from build123d import *

# Parameters (mm, degrees)
BOSS_EXTRU_1_DEPTH             = 4
BOSS_EXTRU_1_DEPTH_BACK        = 4
ESQUISSE3_R                    = 2
ENL_V_MAT_EXTRU_1_DEPTH        = 5
ENL_V_MAT_EXTRU_1_DEPTH_BACK   = 5
BOSS_EXTRU_2_REACH             = 6
BOSS_EXTRU_2_DIRECTION_2_REACH = 6
ENL_V_START                    = -4
ESQUISSE4_W                    = 60
ESQUISSE4_H                    = 3.5
ENL_V_MAT_EXTRU_2_DEPTH        = 5
ENL_V_START_2                  = 9.713229
ESQUISSE7_R                    = 1.5
ENL_V_MAT_EXTRU_4_DEPTH        = 6.063229
CONG_1_R                       = 10
CONG_2_R                       = 2


with BuildPart() as part:
    # Esquisse1 → Boss.-Extru.1 (new body, two sides)
    with BuildSketch(Plane.XY) as boss_extru_1_sk:
        Polygon((-18.056919343, 0.131274222), (-15.479170984, -5.286770941), (18.771312817, -5.286770941), (21.159805355, 1.060426821), (3, 16.8), (-3, 16.8), align=None)
    extrude(amount=BOSS_EXTRU_1_DEPTH)
    extrude(boss_extru_1_sk.sketch, amount=-BOSS_EXTRU_1_DEPTH_BACK)

    # Esquisse3 → Enlèv. mat.-Extru.1 (cut, two sides)
    with BuildSketch(Plane.XY) as enl_v_mat_extru_1_sk:
        with Locations((0, 10.8)):
            Circle(ESQUISSE3_R)
        with Locations((-11.35, 0)):
            Circle(ESQUISSE3_R)
        with Locations((14.35, 0)):
            Circle(ESQUISSE3_R)
    extrude(amount=ENL_V_MAT_EXTRU_1_DEPTH, mode=Mode.SUBTRACT)
    extrude(enl_v_mat_extru_1_sk.sketch, amount=-ENL_V_MAT_EXTRU_1_DEPTH_BACK, mode=Mode.SUBTRACT)

    # Boss.-Extru.2: up to this face of the body (flat: up to its plane)
    boss_extru_2_end = Plane(part.part.faces().sort_by_distance((1.373128785, 3.366991502, 4))[0])
    # Esquisse6 → Boss.-Extru.2 (add, up to the picked face)
    with BuildSketch(Plane.XY, mode=Mode.PRIVATE) as boss_extru_2_sk1:
        Polygon((-9.401505424, 9.713229059), (-30, 9.713229059), (-30, -5.286770941), (-15.479170984, -5.286770941), (-18.056919343, 0.131274222), align=None)
    boss_extru_2_tool1 = split(extrude(boss_extru_2_sk1.sketch, amount=BOSS_EXTRU_2_REACH, mode=Mode.PRIVATE), bisect_by=boss_extru_2_end, keep=Keep.BOTH, mode=Mode.PRIVATE)
    add(boss_extru_2_tool1.solids().sort_by_distance((-22.205202, 2.823075, 0))[0])
    # Esquisse6 → Boss.-Extru.2 (add, up to the picked face)
    with BuildSketch(Plane.XY, mode=Mode.PRIVATE) as boss_extru_2_sk2:
        Polygon((18.771312817, -5.286770941), (30, -5.286770941), (30, 9.713229059), (11.176484802, 9.713229059), (21.159805355, 1.060426821), align=None)
    boss_extru_2_tool2 = split(extrude(boss_extru_2_sk2.sketch, amount=BOSS_EXTRU_2_REACH, mode=Mode.PRIVATE), bisect_by=boss_extru_2_end, keep=Keep.BOTH, mode=Mode.PRIVATE)
    add(boss_extru_2_tool2.solids().sort_by_distance((23.539357, 3.077844, 0))[0])

    # Boss.-Extru.2 direction 2: up to this face of the body (flat: up to its plane)
    boss_extru_2_direction_2_end = Plane(part.part.faces().sort_by_distance((1.373128785, 3.366991502, -4))[0])
    # Esquisse6 → Boss.-Extru.2 direction 2 (add, up to the picked face)
    with BuildSketch(Plane.XY, mode=Mode.PRIVATE) as boss_extru_2_direction_2_sk1:
        Polygon((-9.401505424, 9.713229059), (-30, 9.713229059), (-30, -5.286770941), (-15.479170984, -5.286770941), (-18.056919343, 0.131274222), align=None)
    boss_extru_2_direction_2_tool1 = split(extrude(boss_extru_2_direction_2_sk1.sketch, amount=-BOSS_EXTRU_2_DIRECTION_2_REACH, mode=Mode.PRIVATE), bisect_by=boss_extru_2_direction_2_end, keep=Keep.BOTH, mode=Mode.PRIVATE)
    add(boss_extru_2_direction_2_tool1.solids().sort_by_distance((-22.205202, 2.823075, 0))[0])
    # Esquisse6 → Boss.-Extru.2 direction 2 (add, up to the picked face)
    with BuildSketch(Plane.XY, mode=Mode.PRIVATE) as boss_extru_2_direction_2_sk2:
        Polygon((18.771312817, -5.286770941), (30, -5.286770941), (30, 9.713229059), (11.176484802, 9.713229059), (21.159805355, 1.060426821), align=None)
    boss_extru_2_direction_2_tool2 = split(extrude(boss_extru_2_direction_2_sk2.sketch, amount=-BOSS_EXTRU_2_DIRECTION_2_REACH, mode=Mode.PRIVATE), bisect_by=boss_extru_2_direction_2_end, keep=Keep.BOTH, mode=Mode.PRIVATE)
    add(boss_extru_2_direction_2_tool2.solids().sort_by_distance((23.539357, 3.077844, 0))[0])

    # Esquisse4 → Enlèv. mat.-Extru.2 (cut)
    with BuildSketch(Plane.XY.offset(ENL_V_START)):
        with Locations((0, 5.4)):
            Rectangle(ESQUISSE4_W, ESQUISSE4_H)
    extrude(amount=ENL_V_MAT_EXTRU_2_DEPTH, mode=Mode.SUBTRACT)

    # Esquisse7 → Enlèv. mat.-Extru.4 (cut)
    with BuildSketch(Plane(origin=(0, 0, 0), x_dir=(1, 0, 0), z_dir=(0, 1, 0)).offset(ENL_V_START_2)):
        with Locations((-22, 0)):
            Circle(ESQUISSE7_R)
        with Locations((22, 0)):
            Circle(ESQUISSE7_R)
    extrude(amount=-ENL_V_MAT_EXTRU_4_DEPTH, mode=Mode.SUBTRACT)

    # Congé1
    cong_1_edges = [part.edges().sort_by_distance(p)[0] for p in [
        (30, -5.286770941, 0),
        (-30, -5.286770941, 0),
    ]]
    fillet(cong_1_edges, radius=CONG_1_R)

    # Congé2
    cong_2_edges = [part.edges().sort_by_distance(p)[0] for p in [
        (0, -5.286770941, -4),
        (-26.684598321, -2.724253398, -4),
        (26.684598321, -2.724253398, -4),
        (0, 16.8, -4),
        (-6.200752712, 13.256614529, -4),
        (-19.700752712, 9.713229059, -4),
        (-30, 8.431614529, -4),
        (7.088242401, 13.256614529, -4),
        (20.588242401, 9.713229059, -4),
        (30, 8.431614529, -4),
    ]]
    fillet(cong_2_edges, radius=CONG_2_R)


solid = part.part
Geometry check sheet. Reference: the model listing, model coordinates, mm. A direction names the side the tool comes from. Coordinates: 2 decimals unless noted, no trailing zeros. Loops run counter-clockwise (first coordinate to the right, second up) from the corner with the lowest first, then second, coordinate; pieces in that order, holes last. Notation, with made-up numbers: (16, 48.5) - (26, 48.5) arc R15 cw to (26, 55.5) - close; hole circle Ø9 at (-16, 32). An arc over 180 degrees is marked (long way). Use one line per item in the form item = value. Start each with the question number.
Item 1: Tool access check on faces 5 (the face through (-19.41, 9.14, -3.4)), 6 (the face through (20.08, 9.14, -3.4)), 7 (the face through (20.72, 9.713, 1.042)), 8 (the face through (21.675, 8.071, 1.464)). Record the directions out of +Z, -Z, +X, -X, +Y, -Y that give a thin tool (end or side, any length) a straight path to the whole face; none if there is none.
Item 2: Thickness scan on probe 1 along Y at (x, z) = (-26, 0); probe 2 along Y at (x, z) = (3, 0); probe 3 along Y at (x, z) = (0, -0.5). Record the ranges inside material, lowest first.
Item 3: Section check C-C, the plane z = 2.5. Enter the section's corners in (x, y), and give its area (3 significant figures).
Item 4: Section check D-D, the plane z = -3. Enter the section's corners in (x, y).
Item 5: Mould release check, pull along Y, two halves, no side actions. Record for faces 1 (the face through (-9.503, -0.766, 0.056)), 2 (the face through (6.94, 12.63, -3.4)), 3 (the face through (27, 5, 1)), 4 (the face through (26.99, -2.44, 1.04)): +Y half, -Y half, draft (parallel to the pull), parting line (faces both ways), or undercut.
Item 6: Section check B-B, the plane z = 0. Enter the section's corners in (x, y).
Item 7: Section check A-A, the plane x = 0. Enter the section's corners in (y, z), and give its area (3 significant figures).
Item 8: Gauge pin test, flat ends, axial feed: pin 1 (3 mm diameter, centred on x = -11.5, z = -1.5, fed in from +Y); pin 2 (3 mm diameter, centred on x = -25.5, y = 5.5, fed in from -Z); pin 3 (2 mm diameter, centred on y = 14, z = 0, fed in from +X); pin 4 (3.5 mm diameter, centred on x = 14.35, y = 0, fed in from +Z). Record the tip position at first contact, or that the pin passes through.
Computed:
q1.face_5 = -Z, -X, +Y
q1.face_6 = -Z, +X, +Y
q1.face_7 = +Z, -Z, +X, +Y
q1.face_8 = +Y
q2.probe_1 = -3.29 to 3.65, 7.15 to 9.71
q2.probe_2 = -5.29 to 3.65, 7.15 to 16.8
q2.probe_3 = -5.29 to 3.65, 7.15 to 8.8, 12.8 to 16.8
q3.outline = (-30, 4.71) arc R10 ccw to (-20, -5.29) - (20, -5.29) arc R10 ccw to (30, 4.71) - (30, 9.71) - (11.18, 9.71) - (3, 16.8) - (-3, 16.8) - (-9.4, 9.71) - (-30, 9.71) - close; hole circle Ø4 at (-11.35, 0); hole circle Ø4 at (0, 10.8); hole circle Ø4 at (14.35, 0)
q3.area = 914 mm2
q4.outline = (-29.73, 7.15) - (29.73, 7.15) - (29.73, 9.45) - (11.08, 9.45) - (2.9, 16.53) - (-2.88, 16.53) - (-9.28, 9.45) - (-29.73, 9.45) - close; (-29.67, 3.65) arc R9.73 ccw to (-20, -5.02) - (20, -5.02) arc R9.73 ccw to (29.67, 3.65) - close; hole circle Ø4 at (-11.35, 0); hole circle Ø4 at (0, 10.8); hole circle Ø4 at (14.35, 0)
q5.face_1 = undercut
q5.face_2 = +Y half
q5.face_3 = undercut
q5.face_4 = -Y half
q6.outline = (-30, 7.15) - (-23.5, 7.15) - (-23.5, 9.71) - (-30, 9.71) - close; (-29.94, 3.65) arc R10 ccw to (-20, -5.29) - (20, -5.29) arc R10 ccw to (29.94, 3.65) - close; (-20.5, 7.15) - (20.5, 7.15) - (20.5, 9.71) - (11.18, 9.71) - (3, 16.8) - (-3, 16.8) - (-9.4, 9.71) - (-20.5, 9.71) - close; (23.5, 7.15) - (30, 7.15) - (30, 9.71) - (23.5, 9.71) - close; hole circle Ø4 at (-11.35, 0); hole circle Ø4 at (0, 10.8); hole circle Ø4 at (14.35, 0)
q7.outline = (-5.29, -2) arc R2 ccw to (-3.29, -4) - (3.65, -4) - (3.65, 1) - (7.15, 1) - (7.15, -4) - (8.8, -4) - (8.8, 4) - (-5.29, 4) - close; (12.8, -4) - (14.8, -4) arc R2 ccw to (16.8, -2) - (16.8, 4) - (12.8, 4) - close
q7.area = 125 mm2
q8.pin_1 = 9.71
q8.pin_2 = 1
q8.pin_3 = 7.38
q8.pin_4 = through
